Source: CAD feature listing. Evaluate the final solid. Frame: model axes, mm. A direction names the side the tool comes from. Give positions to 0.01 mm unless a question says otherwise; leave off trailing zeros. Loops run counter-clockwise (first coordinate to the right, second up) from the corner with the lowest first, then second, coordinate; pieces in that order, holes last.
from build123d import *

# Parameters (mm, degrees)
F1_DEPTH = 0.635


with BuildPart() as f1:
    # F0 (on Front) → F1 (new body, symmetric)
    with BuildSketch(Plane.XZ):
        with BuildLine():
            Line((-0.635, 7.47181), (-0.635, 9.50381))
            ThreePointArc((-0.635, 9.50381), (-8.248892, 4.7625), (-8.548041, -4.201979))
            Line((-8.548041, -4.201979), (-6.788277, -3.185979))
            Line((-6.788277, -3.185979), (-6.153277, -4.285831))
            Line((-6.153277, -4.285831), (-7.913041, -5.301831))
            ThreePointArc((-7.913041, -5.301831), (0, -9.525), (7.913041, -5.301831))
            Line((7.913041, -5.301831), (6.153277, -4.285831))
            Line((6.153277, -4.285831), (6.788277, -3.185979))
            Line((6.788277, -3.185979), (8.548041, -4.201979))
            ThreePointArc((8.548041, -4.201979), (8.248892, 4.7625), (0.635, 9.50381))
            Line((0.635, 9.50381), (0.635, 7.47181))
            Line((0.635, 7.47181), (-0.635, 7.47181))
        make_face()
    extrude(amount=F1_DEPTH, both=True)


solid = f1.part
1) Cut plane D-D (x = 3). Return loops of the section in (y, z) (3 decimals), and give its area (3 significant figures).
Checks:
outline: (-0.635, -9.04) - (0.635, -9.04) - (0.635, 9.04) - (-0.635, 9.04) - close
area: 23.0 mm2
2) Ray query, probe 1 along Z at (x, y) = (7.5, -0.25); probe 2 along X at (y, z) = (0.4, -2); probe 3 along X at (y, z) = (-0.2, 8) (3 decimals). Return the intervals inside material, ascending.
Checks:
probe 1: z = -5.87 to -5.06, -3.6 to 5.87
probe 2: x = -9.31 to 9.31
probe 3: x = -5.17 to -0.635, 0.635 to 5.17
3) Contact query for flat-ended pins moving along their axis: P1, Ø0.6, axis at x = 0, y = -0.5, coming from the +Z side; P2, Ø0.6, axis at y = 0, z = 8, coming from the +X side; P3, Ø8, axis at x = 7, z = 7, coming from the +Y side (3 decimals). Output: stop coordinate, or through.
Checks:
P1: stops at z = 7.47
P2: stops at x = 5.61
P3: stops at y = 0.635
4) Cut plane C-C (x = -3.5). Return loops of the section in (y, z) (3 decimals).
Checks:
outline: (-0.635, -8.859) - (0.635, -8.859) - (0.635, 8.859) - (-0.635, 8.859) - close
5) Reachability of faces 1 (the flat face through (-7.021, -0.009, -4.787)), 2 (the flat face through (6.47, -0.01, -3.74)), 3 (the flat face through (7.045, -0.009, -4.801)), 4 (the flat face through (0, -0.635, 0)), 5 (the flat face through (0, 0, 7.472)) from +Z, -Z, +X, -X, +Y, -Y: full face, straight path, thin tool, end or side. Return the list, or none.
Checks:
face 1: -X, +Y, -Y
face 2: +Y, -Y
face 3: +X, +Y, -Y
face 4: +Z, -Z, +X, -X, -Y
face 5: +Z, +Y, -Y
6) Cut plane B-B (x = -6.5). Return loops of the section in (y, z) (3 decimals), and give its area (3 significant figures).
Checks:
outline: (-0.635, -6.962) - (0.635, -6.962) - (0.635, -4.486) - (-0.635, -4.486) - close; (-0.635, -3.685) - (0.635, -3.685) - (0.635, 6.962) - (-0.635, 6.962) - close
area: 16.7 mm2
7) Pull-direction query (X, two-part tool) for faces 6 (the cylindrical face through (-8.18, -0.01, 4.88)), 7 (the flat face through (-6.475, -0.009, -3.728)), 8 (the flat face through (0, 0.635, 0)); classes: released by +X, released by -X, zero draft, split by the parting line, or undercut.
Checks:
face 6: released by -X
face 7: undercut
face 8: zero draft
8) Cut plane A-A (y = 0.1). Return loops of the section in (x, z) (3 decimals).
Checks:
outline: (-8.548, -4.202) - (-6.788, -3.186) - (-6.153, -4.286) - (-7.913, -5.302) arc R9.525 ccw to (7.913, -5.302) - (6.153, -4.286) - (6.788, -3.186) - (8.548, -4.202) arc R9.525 ccw to (0.635, 9.504) - (0.635, 7.472) - (-0.635, 7.472) - (-0.635, 9.504) arc R9.525 ccw to start
